```python
from build123d import *

# Parameters (mm, degrees)
SKETCH1_R           = 3
BOSS_EXTRUDE1_DEPTH = 1
BOSS_EXTRUDE2_DEPTH = 14


with BuildPart() as part:
    # Sketch1 → Boss-Extrude1 (new body)
    with BuildSketch(Plane(origin=(0, 0, 0), x_dir=(0, 1, 0), z_dir=(0, 0, 1))):
        with Locations(Location((0, 0, 0), (0, 0, 270))):
            Circle(SKETCH1_R)
    extrude(amount=BOSS_EXTRUDE1_DEPTH)

    # Sketch2 → Boss-Extrude2 (add)
    with BuildSketch(Plane.XY.offset(1)):
        with BuildLine():
            Line((-0.95, 2.05), (-0.95, 1.15))
            ThreePointArc((-0.95, 1.15), (-1.008578644, 1.008578644), (-1.15, 0.95))
            Line((-1.15, 0.95), (-2.05, 0.95))
            ThreePointArc((-2.05, 0.95), (-2.191421356, 0.891421356), (-2.25, 0.75))
            Line((-2.25, 0.75), (-2.25, -0.75))
            ThreePointArc((-2.25, -0.75), (-2.191421356, -0.891421356), (-2.05, -0.95))
            Line((-2.05, -0.95), (-1.15, -0.95))
            ThreePointArc((-1.15, -0.95), (-1.008578644, -1.008578644), (-0.95, -1.15))
            Line((-0.95, -1.15), (-0.95, -2.05))
            ThreePointArc((-0.95, -2.05), (-0.891421356, -2.191421356), (-0.75, -2.25))
            Line((-0.75, -2.25), (0.75, -2.25))
            ThreePointArc((0.75, -2.25), (0.891421356, -2.191421356), (0.95, -2.05))
            Line((0.95, -2.05), (0.95, -1.15))
            ThreePointArc((0.95, -1.15), (1.008578644, -1.008578644), (1.15, -0.95))
            Line((1.15, -0.95), (2.05, -0.95))
            ThreePointArc((2.05, -0.95), (2.191421356, -0.891421356), (2.25, -0.75))
            Line((2.25, -0.75), (2.25, 0.75))
            ThreePointArc((2.25, 0.75), (2.191421356, 0.891421356), (2.05, 0.95))
            Line((2.05, 0.95), (1.15, 0.95))
            ThreePointArc((1.15, 0.95), (1.008578644, 1.008578644), (0.95, 1.15))
            Line((0.95, 1.15), (0.95, 2.05))
            ThreePointArc((0.95, 2.05), (0.891421356, 2.191421356), (0.75, 2.25))
            Line((0.75, 2.25), (-0.75, 2.25))
            ThreePointArc((-0.75, 2.25), (-0.891421356, 2.191421356), (-0.95, 2.05))
        make_face()
    extrude(amount=BOSS_EXTRUDE2_DEPTH)


solid = part.part
```
The model under review builds one solid part; all positions refer to its coordinate system, in mm. A direction names the side the tool comes from. Coordinates: 2 decimals unless noted, no trailing zeros. Write each loop counter-clockwise with the first axis right and the second up, starting at its lowest first coordinate (ties: lowest second). Pieces come first, ordered by that corner, then holes. Notation, with made-up numbers: (39.5, -3) -> (88.5, -3) arc R29 ccw to (88.5, 36) -> close; hole circle Ø8 at (41.25, -34). An arc over 180 degrees is marked (long way). One line per item, written item: value. Start each with the question number.
Q1. To check wall thickness, follow probe 1 along Y at (x, z) = (0.2, 11.75); probe 2 along Z at (x, y) = (-2.3, -0.2); probe 3 along Y at (x, z) = (-1.3, 7.25). State the ranges of each line that lie inside material, in increasing order.
Q2. For faces 1 (the face through (0.95, 1.6, 7.9)), 2 (the face through (-2.25, 0, 8)), 3 (the face through (2.25, 0, 8)), 4 (the face through (-1.6, 0.95, 7.9)), list the 3-axis set-ups (+Z, -Z, +X, -X, +Y, -Y) from which the entire face can be reached by the end or side of a thin tool; tool diameter is ignored.
Q3. Add section D-D, the plane y = 2.4. Give the boundary of the cut face in (x, z).
Q4. Add section B-B, the plane x = 0. Give the boundary of the cut face in (y, z), then the cut area to 3 significant figures.
Q5. Add section A-A, the plane z = 8.5. Give the boundary of the cut face in (x, y).
Q6. Clearance check with flat-ended pins moving along their axes: P1, Ø0.7, axis at y = 1.5, z = 5.5, coming from the +X side; P2, Ø1.2, axis at y = -0.5, z = 5.5, coming from the +X side; P3, Ø0.7, axis at x = 1.5, z = 7, coming from the +Y side. State where each tip first meets the part, or that it passes through.
Response:
1. probe 1: -2.25 to 2.25
1. probe 2: 0 to 1
1. probe 3: -0.95 to 0.95
2. face 1: +Z, +X, +Y
2. face 2: +Z, -X, +Y, -Y
2. face 3: +Z, +X, +Y, -Y
2. face 4: +Z, -X, +Y
3. outline: (-1.8, 0) -> (1.8, 0) -> (1.8, 1) -> (-1.8, 1) -> close
4. outline: (-3, 0) -> (3, 0) -> (3, 1) -> (2.25, 1) -> (2.25, 15) -> (-2.25, 15) -> (-2.25, 1) -> (-3, 1) -> close
4. area: 69.0 mm²
5. outline: (-2.25, -0.75) arc R0.2 ccw to (-2.05, -0.95) -> (-1.15, -0.95) arc R0.2 cw to (-0.95, -1.15) -> (-0.95, -2.05) arc R0.2 ccw to (-0.75, -2.25) -> (0.75, -2.25) arc R0.2 ccw to (0.95, -2.05) -> (0.95, -1.15) arc R0.2 cw to (1.15, -0.95) -> (2.05, -0.95) arc R0.2 ccw to (2.25, -0.75) -> (2.25, 0.75) arc R0.2 ccw to (2.05, 0.95) -> (1.15, 0.95) arc R0.2 cw to (0.95, 1.15) -> (0.95, 2.05) arc R0.2 ccw to (0.75, 2.25) -> (-0.75, 2.25) arc R0.2 ccw to (-0.95, 2.05) -> (-0.95, 1.15) arc R0.2 cw to (-1.15, 0.95) -> (-2.05, 0.95) arc R0.2 ccw to (-2.25, 0.75) -> close
6. P1: x = 0.95
6. P2: x = 2.25
6. P3: y = 0.95
